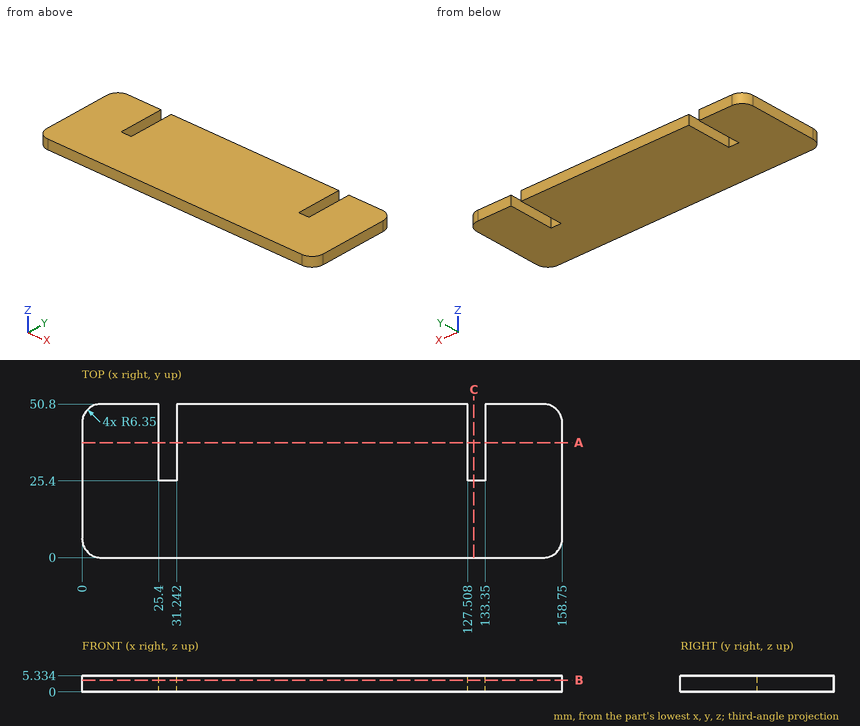
Can you work these out from the drawing? Everything is in mm from the part's minimum corner. Round coordinates to 2 decimals unless told otherwise and drop trailing zeros. Loops run counter-clockwise (first coordinate to the right, second up) from the corner with the lowest first, then second, coordinate; pieces in that order, holes last. Notation, with made-up numbers: (88.5, 33.5) - (117.5, 33.5) arc R12 cw to (117.5, 43.5) - close; hole circle Ø7 at (78.25, 77.5). An arc over 180 degrees is marked (long way). Answer in a Markdown table with one row per item. Add a question column.
(1) I need wall thicknesses on line 1 along X through (y, z) = (41.5, 1.2); line 2 along Y through (x, z) = (131.5, 2.75); line 3 along X through (y, z) = (2, 3.2). Which ranges of each line are inside material? Lowest first, please.
(2) If we section it at A-A (y = 38): Please give me the cut outline in (x, z), plus the area to 3 significant figures.
(3) If we section it at C-C (x = 129.5): Please give me the cut outline in (y, z), plus the area to 3 significant figures.
(4) If we section it at B-B (z = 3.85): Please give me the cut outline in (x, y).
(5) I'm going to push a flat-ended pin straight in: pin 1 (2.5 mm diameter, centred on x = 29.5, z = 3.5, fed in from +Y). Where does the tip first touch, or does it pass through?
Model answer:
| question | item | result |
|---|---|---|
| 1 | line 1 | x = 0 to 25.4, 31.24 to 127.51, 133.35 to 158.75 |
| 1 | line 2 | y = 0 to 25.4 |
| 1 | line 3 | x = 1.72 to 157.03 |
| 2 | outline | (0, 0) - (25.4, 0) - (25.4, 5.33) - (0, 5.33) - close; (31.24, 0) - (127.51, 0) - (127.51, 5.33) - (31.24, 5.33) - close; (133.35, 0) - (158.75, 0) - (158.75, 5.33) - (133.35, 5.33) - close |
| 2 | area | 784 mm² |
| 3 | outline | (0, 0) - (25.4, 0) - (25.4, 5.33) - (0, 5.33) - close |
| 3 | area | 135 mm² |
| 4 | outline | (0, 6.35) arc R6.35 ccw to (6.35, 0) - (152.4, 0) arc R6.35 ccw to (158.75, 6.35) - (158.75, 44.45) arc R6.35 ccw to (152.4, 50.8) - (133.35, 50.8) - (133.35, 25.4) - (127.51, 25.4) - (127.51, 50.8) - (31.24, 50.8) - (31.24, 25.4) - (25.4, 25.4) - (25.4, 50.8) - (6.35, 50.8) arc R6.35 ccw to (0, 44.45) - close |
| 5 | pin 1 | stops at y = 25.4 |
